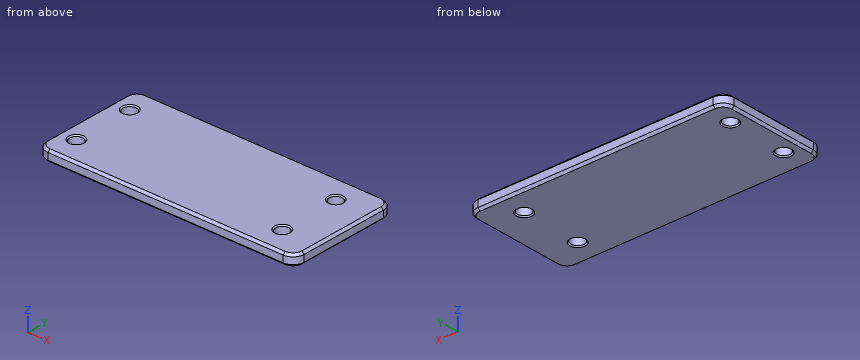
```python
from build123d import *

# Parameters (mm, degrees)
F0_R     = 6
F1_DEPTH = 10
F2_SIZE  = 2
F3_SIZE  = 2
F4_SIZE  = 1
F5_SIZE  = 1


with BuildPart() as f1:
    # F0 (on Top) → F1 (new body)
    with BuildSketch(Plane.XY):
        with BuildLine():
            ThreePointArc((115, 40), (112.071068, 47.071068), (105, 50))
            Line((105, 50), (-105, 50))
            ThreePointArc((-105, 50), (-112.071068, 47.071068), (-115, 40))
            Line((-115, 40), (-115, -40))
            ThreePointArc((-115, -40), (-112.071068, -47.071068), (-105, -50))
            Line((-105, -50), (105, -50))
            ThreePointArc((105, -50), (112.071068, -47.071068), (115, -40))
            Line((115, -40), (115, 40))
        make_face()
        with Locations((-100, -27)):
            Circle(F0_R, mode=Mode.SUBTRACT)
        with Locations((84, -27)):
            Circle(F0_R, mode=Mode.SUBTRACT)
        with Locations((-100, 27)):
            Circle(F0_R, mode=Mode.SUBTRACT)
        with Locations((84, 27)):
            Circle(F0_R, mode=Mode.SUBTRACT)
    extrude(amount=F1_DEPTH)

    # F2
    f2_edges = [f1.edges().sort_by_distance(p)[0] for p in [
        (0, -50, 10),
    ]]
    chamfer(f2_edges, length=F2_SIZE)

    # F3
    f3_edges = [f1.edges().sort_by_distance(p)[0] for p in [
        (0, -50, 0),
    ]]
    chamfer(f3_edges, length=F3_SIZE)

    # F4
    f4_edges = [f1.edges().sort_by_distance(p)[0] for p in [
        (-106, -27, 10),
        (-106, 27, 10),
        (78, 27, 10),
        (78, -27, 10),
    ]]
    chamfer(f4_edges, length=F4_SIZE)

    # F5
    f5_edges = [f1.edges().sort_by_distance(p)[0] for p in [
        (78, -27, 0),
        (78, 27, 0),
        (-106, -27, 0),
        (-106, 27, 0),
    ]]
    chamfer(f5_edges, length=F5_SIZE)


solid = f1.part
```
Geometry check sheet. Reference: the model listing, model coordinates, mm. Coordinates: 2 decimals unless noted, no trailing zeros. Order: outer loops, then holes, each group sorted by start corner. A loop starts at its lowest first (then second) coordinate and runs counter-clockwise, first axis right, second up. Notation, with made-up numbers: M 15.25,57.5 L 52.25,57.5 A29 ccw 52.25,93.5 Z; hole C 70,-37 d2. An arc over 180 degrees is marked long. Answer as a JSON object with one key per item and string values.
Q1. Cross-section at C-C on x = -100. Record the cut outline in (y, z).
Results are:
{"outline": "M -50,2 L -48,0 L -34,0 L -33,1 L -33,9 L -34,10 L -48,10 L -50,8 Z; M -21,1 L -20,0 L 20,0 L 21,1 L 21,9 L 20,10 L -20,10 L -21,9 Z; M 33,1 L 34,0 L 48,0 L 50,2 L 50,8 L 48,10 L 34,10 L 33,9 Z"}
Q2. Depth check by flat-ended pin: pin 1 Ø9.5 at (x, y) = (-100, -27) entering from +Z. Enter the tip coordinate at first touch or a pass-through.
Results are:
{"pin 1": "passes through"}
Q3. Scan lines: line 1 (Y direction, x = 84, z = 4); line 2 (Y direction, x = -104.5, z = 5); line 3 (X direction, y = -28, z = 4). Record each from-to range of solid material in increasing order.
Results are:
{"line 1": "y = -50 to -33, -21 to 21, 33 to 50", "line 2": "y = -50 to -30.97, -23.03 to 23.03, 30.97 to 50", "line 3": "x = -115 to -105.92, -94.08 to 78.08, 89.92 to 115"}
Q4. Cross-section at A-A on y = -27. Record the cut outline in (x, z).
Results are:
{"outline": "M -115,2 L -113,0 L -107,0 L -106,1 L -106,9 L -107,10 L -113,10 L -115,8 Z; M -94,1 L -93,0 L 77,0 L 78,1 L 78,9 L 77,10 L -93,10 L -94,9 Z; M 90,1 L 91,0 L 113,0 L 115,2 L 115,8 L 113,10 L 91,10 L 90,9 Z"}
Q5. Cross-section at B-B on z = 6.25. Record the cut outline in (x, y).
Results are:
{"outline": "M -115,-40 A10 ccw -105,-50 L 105,-50 A10 ccw 115,-40 L 115,40 A10 ccw 105,50 L -105,50 A10 ccw -115,40 Z; hole C -100,-27 d12; hole C -100,27 d12; hole C 84,-27 d12; hole C 84,27 d12"}
